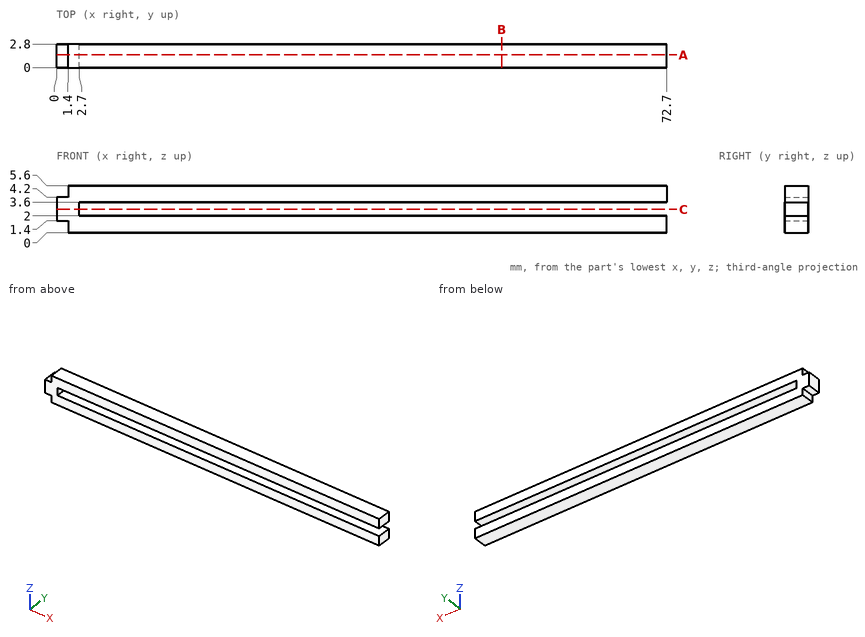
The figure shows three views and two pictorial views of one solid part (mm, origin at its lowest corner). Answer the questions. Give positions to 0.01 mm unless a question says otherwise; leave off trailing zeros. Order: outer loops, then holes, each group sorted by start corner. A loop starts at its lowest first (then second) coordinate and runs counter-clockwise, first axis right, second up. Notation, with made-up numbers: (-32, 11) -> (-13, 11) arc R32 cw to (-13, 38) -> close; hole circle Ø8 at (88, -9.75). An arc over 180 degrees is marked (long way). Write each question's results on one line, items separated by ' | '.
Q1. The part is cut by section A-A, the plane y = 1.5. Give the vertices of the cut face in (x, z), and give its area (3 significant figures).
Checked values:
outline: (0, 1.4) -> (1.4, 1.4) -> (1.4, 0) -> (72.7, 0) -> (72.7, 2) -> (2.7, 2) -> (2.7, 3.6) -> (72.7, 3.6) -> (72.7, 5.6) -> (1.4, 5.6) -> (1.4, 4.2) -> (0, 4.2) -> close | area: 291 mm^2
Q2. Straight lines are drawn through the part: probe 1 along Z at (x, y) = (60.5, 1.25); probe 2 along X at (y, z) = (1.85, 3.25); probe 3 along X at (y, z) = (1.4, 4.25). For each, find the intervals that lie inside material, in ascending order. Write a range as from..to.
Checked values:
probe 1: z = 0..2, 3.6..5.6 | probe 2: x = 0..2.7 | probe 3: x = 1.4..72.7
Q3. The part is cut by section C-C, the plane z = 2.75. Give the vertices of the cut face in (x, y).
Checked values:
outline: (0, 0) -> (2.7, 0) -> (2.7, 2.8) -> (0, 2.8) -> close
Q4. Each of these flat-tipped pins is pushed along its axis until it touches: P1, Ø1.5, axis at y = 1.5, z = 0.5, coming from the -X side; P2, Ø1.5, axis at x = 0.5, y = 1, coming from the +Z side; P3, Ø0.7, axis at x = 0.5, y = 1, coming from the -Z side. Where does it stop, or does it pass through?
Checked values:
P1: stops at x = 1.4 | P2: stops at z = 4.2 | P3: stops at z = 1.4
Q5. The part is cut by section B-B, the plane x = 53. Give the vertices of the cut face in (y, z), and give its area (3 significant figures).
Checked values:
outline: (0, 0) -> (2.8, 0) -> (2.8, 2) -> (0, 2) -> close; (0, 3.6) -> (2.8, 3.6) -> (2.8, 5.6) -> (0, 5.6) -> close | area: 11.2 mm^2
